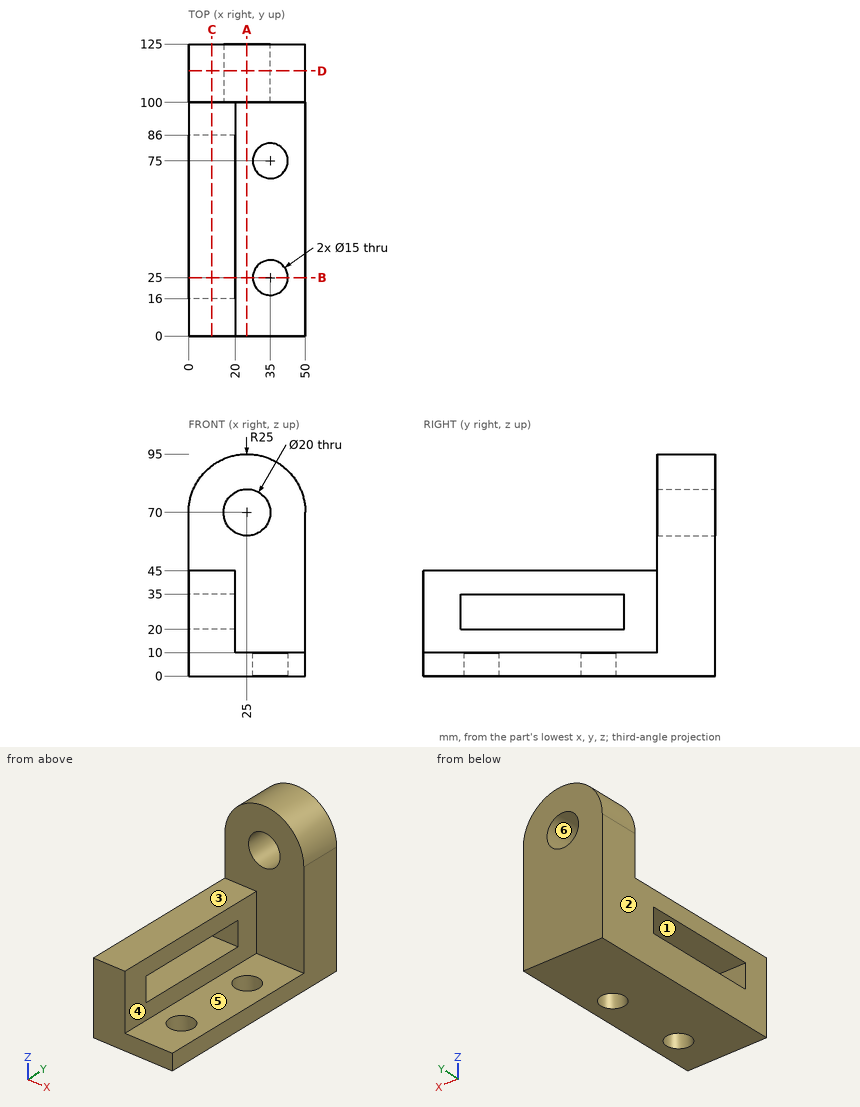
Print and shaded views of the part. All mm, measured from the part's lowest x, y and z. A direction names the side the tool comes from. Coordinates: 2 decimals unless noted, no trailing zeros. Write each loop counter-clockwise with the first axis right and the second up, starting at its lowest first coordinate (ties: lowest second). Pieces come first, ordered by that corner, then holes. Notation, with made-up numbers: (16.25, -16.5) -> (70.25, -16.5) arc R15 cw to (70.25, -8.5) -> close; hole circle Ø6 at (13, 15). An arc over 180 degrees is marked (long way). Use CSV: the item, a comma, the result in double quotes. Start each with the question number.
Q1. 3-axis set-ups, long thin cutter, end or side, ignore diameter. For the marked faces 1, 2 and 3: which of +Z, -Z, +X, -X, +Y, -Y reach the whole face in a straight line?
Q2. Cut at B-B, the plane y = 25. List the corners of the cut face in (x, z).
Q3. Cut at D-D, the plane y = 113.5. List the corners of the cut face in (x, z), then the cut area to 3 significant figures.
Q4. Cut at A-A, the plane x = 25. List the corners of the cut face in (y, z).
Q5. Cut at C-C, the plane x = 10. List the corners of the cut face in (y, z), then the cut area to 3 significant figures.
Q6. Flat gauge pins, fed straight in: pin 1 Ø2 at (x, y) = (37, 110) entering from -Z; pin 2 Ø16 at (x, y) = (7, 69.5) entering from +Z; pin 3 Ø24 at (x, y) = (35, 25) entering from +Z; pin 4 Ø3 at (x, y) = (7.5, 99.5) entering from +Z. Where does each tip first touch, or does it go through?
Q7. Drill centre lines: probe 1 along Y at (x, z) = (35, 8); probe 2 along Z at (x, y) = (25, 106.5); probe 3 along Z at (x, y) = (15, 19.5). Where is each one in solid material? Low to high.
Q8. Pull direction Z, two halves, no side cores. Call the marked faces 4, 5 and 6: released by +Z, released by -Z, zero draft, split by the parting line, or undercut.
Checked values:
1,face 1,"+X, -X"
1,face 2,"+Z, -Z, -X, +Y, -Y"
1,face 3,"+Z, +X, -X, -Y"
2,outline,"(0, 0) -> (27.5, 0) -> (27.5, 10) -> (20, 10) -> (20, 20) -> (0, 20) -> close; (0, 35) -> (20, 35) -> (20, 45) -> (0, 45) -> close; (42.5, 0) -> (50, 0) -> (50, 10) -> (42.5, 10) -> close"
3,outline,"(0, 0) -> (50, 0) -> (50, 70) arc R25 ccw to (0, 70) -> close; hole circle Ø20 at (25, 70)"
3,area,"4,170 mm²"
4,outline,"(0, 0) -> (125, 0) -> (125, 60) -> (100, 60) -> (100, 10) -> (0, 10) -> close; (100, 80) -> (125, 80) -> (125, 95) -> (100, 95) -> close"
5,outline,"(0, 0) -> (125, 0) -> (125, 90) -> (100, 90) -> (100, 45) -> (0, 45) -> close; hole (16, 20) -> (86, 20) -> (86, 35) -> (16, 35) -> close"
5,area,"5,700 mm²"
6,pin 1,"stops at z = 0"
6,pin 2,"stops at z = 45"
6,pin 3,"stops at z = 10"
6,pin 4,"stops at z = 89.14"
7,probe 1,"y = 0 to 17.5, 32.5 to 67.5, 82.5 to 125"
7,probe 2,"z = 0 to 60, 80 to 95"
7,probe 3,"z = 0 to 20, 35 to 45"
8,face 4,"zero draft"
8,face 5,"released by +Z"
8,face 6,"undercut"
